Work out the finished part from the listing and answer in its coordinate system (mm). A direction names the side the tool comes from. Give positions to 0.01 mm unless a question says otherwise; leave off trailing zeros. Write each loop counter-clockwise with the first axis right and the second up, starting at its lowest first coordinate (ties: lowest second). Pieces come first, ordered by that corner, then holes.
1) Find section C-C (y = 1.4). Determine the outline of the cut face in (x, z) (3 decimals), plus the area to 3 significant figures.
2) Find section B-B (z = 29.5). Determine the outline of the cut face in (x, y).
3) A tool of negligible diameter and unlimited length cuts with its end or side. For faces 4 (the face through (3.467, 1.264, -40.443)), 5 (the face through (0.184, 1.236, -52.747)), 6 (the face through (-3.494, 1.264, 40.526)), from which of +Z, -Z, +X, -X, +Y, -Y can it reach the whole face along a straight path? Write none if from no direction.
4) Given pin 1 Ø1 at (y, z) = (1, -33) entering from +X; pin 2 Ø1 at (y, z) = (1.5, -18) entering from -X; pin 3 Ø1 at (x, z) = (4.5, -7) entering from -Y, each flat-ended and moving along its own axis, determine where each tip first touches the part or whether it passes through.
5) Straight lines are drawn through the part: probe 1 along Z at (x, y) = (0, 1.1); probe 2 along X at (y, z) = (1.1, -46.75); probe 3 along Z at (x, y) = (-1, 0.6). For each, find the intervals that lie inside material, in ascending order.
6) Find section A-A (x = 0). Determine the outline of the cut face in (y, z), plus the area to 3 significant figures.
7) Determine the mould class of faces 1 (the face through (-3, 1, -1)), 2 (the face through (0, 2.5, -1)), 3 (the face through (-3.467, 1.264, -40.443)) for opening direction Z: pulls with the +Z half, pulls with the -Z half, needs draft (parallel to the pull), parting line crosses it, or undercut.
```python
from build123d import *

# Parameters (mm, degrees)
SKETCH1_R           = 2
BOSS_EXTRUDE1_DEPTH = 2.5
FILLET1_R           = 10
FILLET2_R           = 0.25


with BuildPart() as part:
    # Sketch1 → Boss-Extrude1 (new body)
    with BuildSketch(Plane(origin=(0, 0, 0), x_dir=(1, 0, 0), z_dir=(0, 1, 0))):
        with BuildLine():
            ThreePointArc((-3, -41.553847577), (0, -52.75), (3, -41.553847577))
            Line((3, -41.553847577), (3, 41.553847577))
            ThreePointArc((3, 41.553847577), (0, 52.75), (-3, 41.553847577))
            Line((-3, 41.553847577), (-3, -41.553847577))
        make_face()
        with Locations((0, -46.75)):
            Circle(SKETCH1_R, mode=Mode.SUBTRACT)
        with Locations((0, 46.75)):
            Circle(SKETCH1_R, mode=Mode.SUBTRACT)
    extrude(amount=BOSS_EXTRUDE1_DEPTH)

    # Fillet1
    fillet1_edges = [part.edges().sort_by_distance(p)[0] for p in [
        (-3, 1.25, 41.553847577),
        (-3, 1.25, -41.553847577),
        (3, 1.25, -41.553847577),
        (3, 1.25, 41.553847577),
    ]]
    fillet(fillet1_edges, radius=FILLET1_R)

    # Fillet2
    fillet2_edges = [part.edges().sort_by_distance(p)[0] for p in [
        (0, 0, 52.75),
        (0, 2.5, 52.75),
        (-3, 0, 0),
        (-3, 2.5, 0),
        (0, 0, -52.75),
        (0, 2.5, -52.75),
        (3, 0, 0),
        (3, 2.5, 0),
        (-3.480283618, 0, 40.484483125),
        (-3.480283618, 2.5, 40.484483125),
        (-3.480283618, 0, -40.484483125),
        (-3.480283618, 2.5, -40.484483125),
        (3.480283618, 0, -40.484483125),
        (3.480283618, 2.5, -40.484483125),
        (3.480283618, 0, 40.484483125),
        (3.480283618, 2.5, 40.484483125),
    ]]
    fillet(fillet2_edges, radius=FILLET2_R)


solid = part.part
```
Results:
1. outline: (-4.875, -43.252) arc R6 ccw (long way) to (4.875, -43.252) arc R10 cw to (3, -37.423) - (3, 37.423) arc R10 cw to (4.875, 43.252) arc R6 ccw (long way) to (-4.875, 43.252) arc R10 cw to (-3, 37.423) - (-3, -37.423) arc R10 cw to start; hole circle Ø4 at (0, -46.75); hole circle Ø4 at (0, 46.75)
1. area: 700 mm2
2. outline: (-3, 0.25) arc R0.25 ccw to (-2.75, 0) - (2.75, 0) arc R0.25 ccw to (3, 0.25) - (3, 2.25) arc R0.25 ccw to (2.75, 2.5) - (-2.75, 2.5) arc R0.25 ccw to (-3, 2.25) - close
3. face 4: +X, +Y, -Y
3. face 5: +Y, -Y
3. face 6: -X, +Y, -Y
4. pin 1: stops at x = 3
4. pin 2: stops at x = -3
4. pin 3: passes through
5. probe 1: z = -52.75 to -48.75, -44.75 to 44.75, 48.75 to 52.75
5. probe 2: x = -6 to -2, 2 to 6
5. probe 3: z = -52.67 to -48.48, -45.02 to 45.02, 48.48 to 52.67
6. outline: (0, -52.5) arc R0.25 ccw to (0.25, -52.75) - (2.25, -52.75) arc R0.25 ccw to (2.5, -52.5) - (2.5, -48.75) - (0, -48.75) - close; (0, -44.75) - (2.5, -44.75) - (2.5, 44.75) - (0, 44.75) - close; (0, 48.75) - (2.5, 48.75) - (2.5, 52.5) arc R0.25 ccw to (2.25, 52.75) - (0.25, 52.75) arc R0.25 ccw to (0, 52.5) - close
6. area: 244 mm2
7. face 1: undercut
7. face 2: needs draft
7. face 3: undercut
